Part print with two shaded views. Sizes in mm from the minimum x, y, z corner. A direction names the side the tool comes from. Give positions to 0.01 mm unless a question says otherwise; leave off trailing zeros. Loops run counter-clockwise (first coordinate to the right, second up) from the corner with the lowest first, then second, coordinate; pieces in that order, holes last. Notation, with made-up numbers: M 3.25,70.5 L 13.25,70.5 A20 cw 13.25,90.5 Z; hole C -25,82.5 d11. An arc over 180 degrees is marked long. Answer as a JSON object with one key per item and string values. Group by question number.
1. 3-axis set-ups, long thin cutter, end or side, ignore diameter. For the marked faces 1 and 2: which of +Z, -Z, +X, -X, +Y, -Y reach the whole face in a straight line?
2. Drop flat-ended pins along their axis: pin 1 Ø8 at (x, y) = (22.5, 12) entering from +Z; pin 2 Ø3.5 at (x, y) = (15.14, 7.75) entering from +Z. Give the stop position or say it passes through.
3. Drill centre lines: line 1 along Y through (x, z) = (22.5, 2.05); line 2 along Z through (x, y) = (5, 12); line 3 along X through (y, z) = (8, 5.5). Where is each one in solid material? Low to high. Write a range as [from, to].
4. Slice it at C-C (y = 7.75). List the corners of the cut face in (x, z), then the cut area to 3 significant figures.
5. Slice it at A-A (y = 12). List the corners of the cut face in (x, z), then the cut area to 3 significant figures.
6. Slice it at D-D (x = 40). List the corners of the cut face in (y, z).
7. Slice it at B-B (x = 22.5). List the corners of the cut face in (y, z).
8. Mould opens along Y. For the marked faces 3, 4, 5 and 6 say: released by +Y, released by -Y, zero draft, split by the parting line, or undercut.
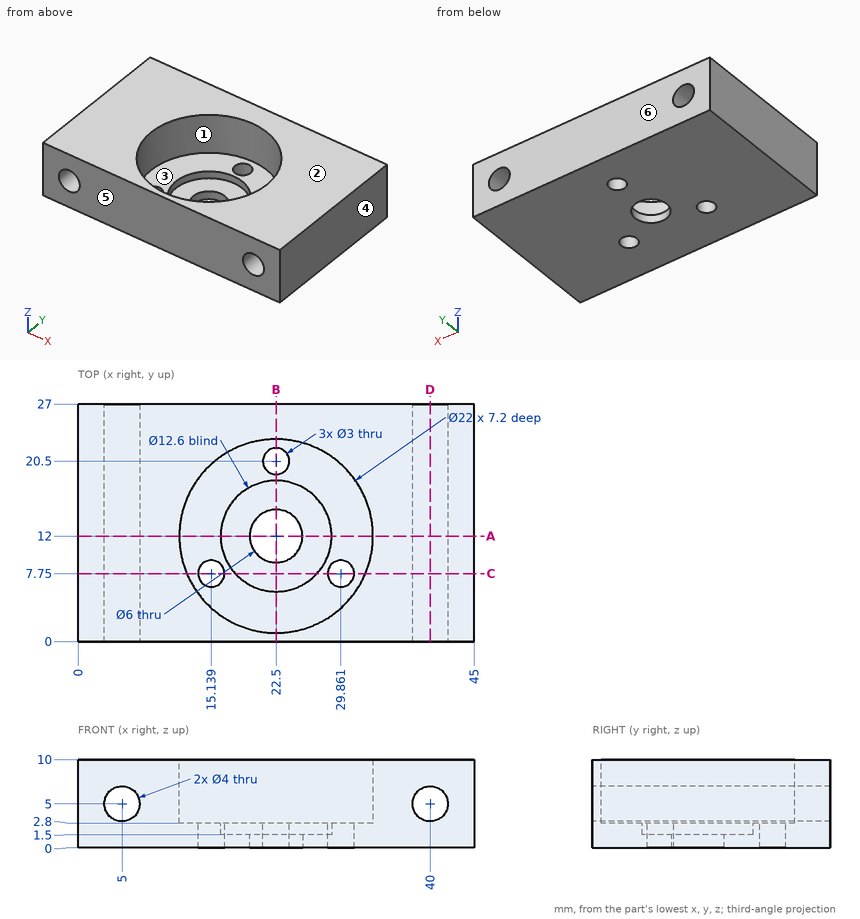
Established:
{
 "1": {"face 1": "+Z", "face 2": "+Z, +X, -X, +Y, -Y"},
 "2": {"pin 1": "stops at z = 1.5", "pin 2": "stops at z = 2.8"},
 "3": {"line 1": "y = [0, 5.7], [18.3, 19], [22, 27]", "line 2": "z = [0, 3], [7, 10]", "line 3": "x = [0, 3.06], [6.94, 12.25], [32.75, 38.06], [41.94, 45]"},
 "4": {"outline": "M 0,0 L 13.64,0 L 13.64,2.8 L 12.35,2.8 L 12.35,10 L 0,10 Z; M 16.64,0 L 28.36,0 L 28.36,2.8 L 27.15,2.8 L 27.15,1.5 L 17.85,1.5 L 17.85,2.8 L 16.64,2.8 Z; M 31.36,0 L 45,0 L 45,10 L 32.65,10 L 32.65,2.8 L 31.36,2.8 Z; hole C 5,5 d4; hole C 40,5 d4", "area": "250 mm^2"},
 "5": {"outline": "M 0,0 L 19.5,0 L 19.5,1.5 L 16.2,1.5 L 16.2,2.8 L 11.5,2.8 L 11.5,10 L 0,10 Z; M 25.5,0 L 45,0 L 45,10 L 33.5,10 L 33.5,2.8 L 28.8,2.8 L 28.8,1.5 L 25.5,1.5 Z; hole C 5,5 d4; hole C 40,5 d4", "area": "241 mm^2"},
 "6": {"outline": "M 0,0 L 27,0 L 27,3 L 0,3 Z; M 0,7 L 27,7 L 27,10 L 0,10 Z"},
 "7": {"outline": "M 0,0 L 9,0 L 9,1.5 L 5.7,1.5 L 5.7,2.8 L 1,2.8 L 1,10 L 0,10 Z; M 15,0 L 19,0 L 19,2.8 L 18.3,2.8 L 18.3,1.5 L 15,1.5 Z; M 22,0 L 27,0 L 27,10 L 23,10 L 23,2.8 L 22,2.8 Z"},
 "8": {"face 3": "undercut", "face 4": "zero draft", "face 5": "released by -Y", "face 6": "released by +Y"}
}
